Geometry check sheet. Reference: the model listing, model coordinates, mm. A direction names the side the tool comes from. Give positions to 0.01 mm unless a question says otherwise; leave off trailing zeros. Write each loop counter-clockwise with the first axis right and the second up, starting at its lowest first coordinate (ties: lowest second). Pieces come first, ordered by that corner, then holes. Notation, with made-up numbers: (-35, 23) -> (24, 23) arc R20 ccw to (24, 59) -> close; hole circle Ø4 at (-10.5, -3.75). An arc over 180 degrees is marked (long way). One line per item, written item: value.
from build123d import *

# Parameters (mm, degrees)
EXTRUDE_1_DEPTH          = 4
CUT_EXTRUDE_1_REACH      = 32.282
SKETCH_2_R               = 2
CUT_EXTRUDE_2_DEPTH      = 31.282007859
CUT_EXTRUDE_2_DEPTH_BACK = 31.282007859
SKETCH_3_R               = 2


with BuildPart() as part:
    # 草图1 → 凸台-拉伸1 (new, symmetric)
    with BuildSketch(Plane(origin=(0, 0, 0), x_dir=(0, 0, -1), z_dir=(1, 0, 0))):
        Polygon((-15, 0), (-15, -5), (-5, -5), (-5, -26), (5, -26), (5, -5), (15, -5), (15, 0), (0, 0), align=None)
    extrude(amount=EXTRUDE_1_DEPTH, both=True)

    # 草图2 → 切除-拉伸1 (cut, up to next)
    with BuildSketch(Plane(origin=(0, 0, 0), x_dir=(1, 0, 0), z_dir=(0, 1, 0)), mode=Mode.PRIVATE) as cut_extrude_1_sk1:
        with Locations(Location((0, 10, 0), (0, 0, 270))):
            Circle(SKETCH_2_R)
    cut_extrude_1_tool1 = extrude(cut_extrude_1_sk1.sketch, amount=-CUT_EXTRUDE_1_REACH, mode=Mode.PRIVATE) & part.part
    # 草图2 → 切除-拉伸1 (cut, up to next)
    with BuildSketch(Plane(origin=(0, 0, 0), x_dir=(1, 0, 0), z_dir=(0, 1, 0)), mode=Mode.PRIVATE) as cut_extrude_1_sk2:
        with Locations(Location((0, -10, 0), (0, 0, 270))):
            Circle(SKETCH_2_R)
    cut_extrude_1_tool2 = extrude(cut_extrude_1_sk2.sketch, amount=-CUT_EXTRUDE_1_REACH, mode=Mode.PRIVATE) & part.part
    add(cut_extrude_1_tool1.solids().sort_by_distance((0, 0, -10))[0], mode=Mode.SUBTRACT)
    add(cut_extrude_1_tool2.solids().sort_by_distance((0, 0, 10))[0], mode=Mode.SUBTRACT)

    # 草图3 → 切除-拉伸2 (cut, two sides: drawn at the far end of the back side and taken through both)
    with BuildSketch(Plane.XY.offset(-CUT_EXTRUDE_2_DEPTH_BACK)):
        with Locations(Location((0, -20, 0), (0, 0, 270))):
            Circle(SKETCH_3_R)
    extrude(amount=CUT_EXTRUDE_2_DEPTH + CUT_EXTRUDE_2_DEPTH_BACK, mode=Mode.SUBTRACT)


solid = part.part
1) Mould release check, pull along X, two halves, no side actions. Record for faces 1 (the cylindrical face through (-1.2, -18.4, -0.1)), 2 (the flat face through (0, -3, -15)), 3 (the flat face through (-4, -10, 0)): released by +X, released by -X, zero draft, split by the parting line, or undercut.
Verdict:
face 1: undercut
face 2: zero draft
face 3: released by -X
2) Sectioned sample at A-A on y = -20. Record the cut outline in (x, z).
Verdict:
outline: (-4, -5) -> (-2, -5) -> (-2, 5) -> (-4, 5) -> close; (2, -5) -> (4, -5) -> (4, 5) -> (2, 5) -> close
3) Scan lines: probe 1 along X at (y, z) = (-3.8, 10); probe 2 along Y at (x, z) = (0, -2.5); probe 3 along Z at (x, y) = (1.5, -3.75). Record each from-to range of solid material in increasing order.
Verdict:
probe 1: -4 to -2, 2 to 4
probe 2: -26 to -22, -18 to 0
probe 3: -15 to -11.32, -8.68 to 8.68, 11.32 to 15
4) Sectioned sample at B-B on z = -10. Record the cut outline in (x, y), plus the area to 3 significant figures.
Verdict:
outline: (-4, -5) -> (-2, -5) -> (-2, 0) -> (-4, 0) -> close; (2, -5) -> (4, -5) -> (4, 0) -> (2, 0) -> close
area: 20.0 mm^2
5) Tool access check on faces 4 (the flat face through (0, -16, -5)), 5 (the flat face through (2, -5, 11)), 6 (the cylindrical face through (-1.2, -2.5, 8.4)). Record the directions out of +Z, -Z, +X, -X, +Y, -Y that give a thin tool (end or side, any length) a straight path to the whole face; none if there is none.
Verdict:
face 4: -Z, +X, -X, -Y
face 5: +Z, +X, -X, -Y
face 6: +Y, -Y
6) Sectioned sample at C-C on x = 1. Record the cut outline in (y, z), plus the area to 3 significant figures.
Verdict:
outline: (-26, -5) -> (-21.73, -5) -> (-21.73, 5) -> (-26, 5) -> close; (-18.27, -5) -> (-5, -5) -> (-5, -8.27) -> (0, -8.27) -> (0, 8.27) -> (-5, 8.27) -> (-5, 5) -> (-18.27, 5) -> close; (-5, -15) -> (0, -15) -> (0, -11.73) -> (-5, -11.73) -> close; (-5, 11.73) -> (0, 11.73) -> (0, 15) -> (-5, 15) -> close
area: 291 mm^2
7) Depth check by flat-ended pin: pin 1 Ø2.5 at (x, y) = (2, -17.5) entering from -Z; pin 2 Ø5 at (y, z) = (-18.5, 8) entering from -X (3 decimals); pin 3 Ø4 at (x, y) = (0, -17.5) entering from +Z. Enter the tip coordinate at first touch or a pass-through.
Verdict:
pin 1: z = -5
pin 2: through
pin 3: z = 5
8) Sectioned sample at D-D on z = 2.75. Record the cut outline in (x, y).
Verdict:
outline: (-4, -26) -> (4, -26) -> (4, 0) -> (-4, 0) -> close; hole circle Ø4 at (0, -20)
